Can you work these out from the drawing? Everything is in mm from the part's minimum corner. A direction names the side the tool comes from. Coordinates: 2 decimals unless noted, no trailing zeros. Order: outer loops, then holes, each group sorted by start corner. A loop starts at its lowest first (then second) coordinate and runs counter-clockwise, first axis right, second up. Notation, with made-up numbers: (19.25, 31.25) -> (56.25, 31.25) arc R19 cw to (56.25, 40.25) -> close; hole circle Ø3 at (16, 14). An arc over 180 degrees is marked (long way). Use a Markdown table: item, result. Add a question column.
1) If I drill on L1, parallel to Y at x = 70.8, z = 3.05; L2, parallel to Y at x = 70, z = 2; L3, parallel to Y at x = 69.5, z = 35.5, over which ranges is the centre line in solid material (lowest first)? Write a range as [from, to].
2) Which directions (+Z, -Z, +X, -X, +Y, -Y) give clear straight access to the entire face, cutting with the end or side of a thin tool? Please do the marked faces 1 and 2.
3) If we section it at C-C (x = 108): Write out the boundary of the cut face in (y, z), plus the area to 3 significant figures.
4) If we section it at D-D (z = 26): Write out the boundary of the cut face in (x, y).
5) If we section it at B-B (y = 10): Write out the boundary of the cut face in (x, z), plus the area to 3 significant figures.
6) If we section it at A-A (x = 70.8): Write out the boundary of the cut face in (y, z), plus the area to 3 significant figures.
7) Will these pins go through, and if not, where does the flat tip stop? pin 1 Ø7.5 at (x, y) = (113.79, 27.81) entering from +Z; pin 2 Ø4 at (x, y) = (10, 70.8) entering from -Z; pin 3 Ø10 at (x, z) = (65.5, 14.5) entering from -Y; pin 4 Ø10 at (y, z) = (80.5, 36) entering from -X.
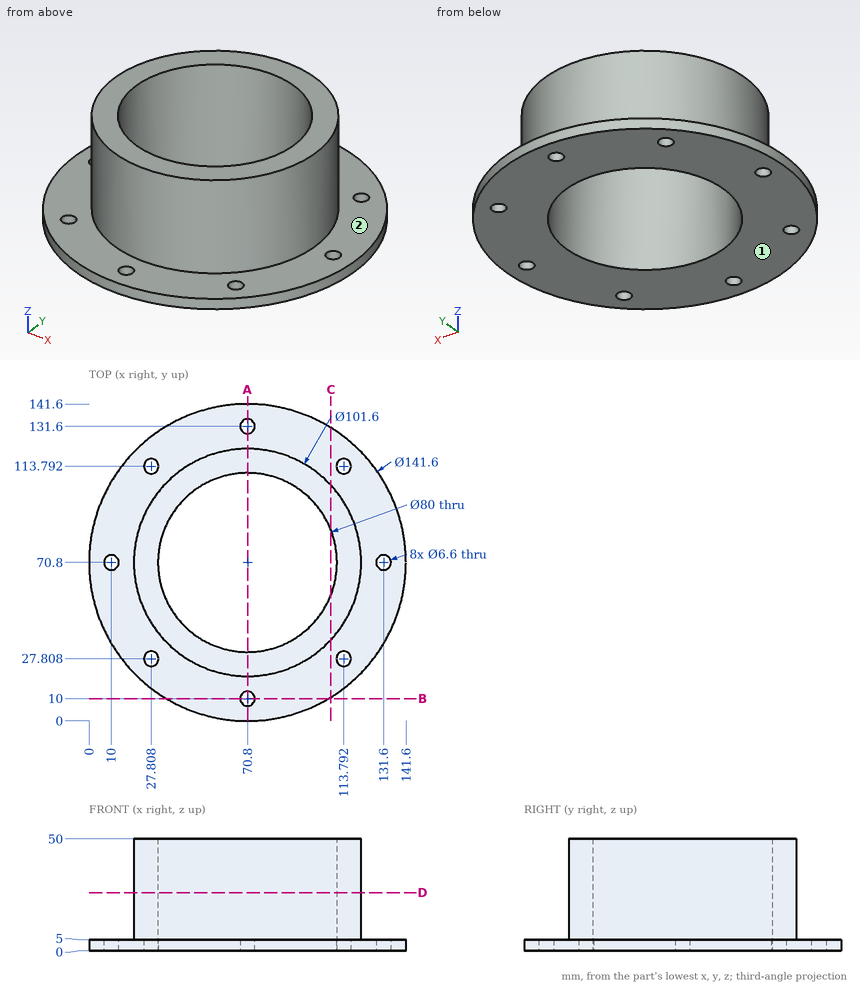
Answer sheet:
| question | item | result |
|---|---|---|
| 1 | L1 | [0, 6.7], [13.3, 30.8], [110.8, 128.3], [134.9, 141.6] |
| 1 | L2 | [0, 6.8], [13.2, 30.81], [110.79, 128.4], [134.8, 141.6] |
| 1 | L3 | [20.02, 30.82], [110.78, 121.58] |
| 2 | face 1 | -Z, +X, -X, +Y, -Y |
| 2 | face 2 | +Z |
| 3 | outline | (10.56, 0) -> (56.1, 0) -> (56.1, 50) -> (36.21, 50) -> (36.21, 5) -> (10.56, 5) -> close; (85.5, 0) -> (131.04, 0) -> (131.04, 5) -> (105.39, 5) -> (105.39, 50) -> (85.5, 50) -> close |
| 3 | area | 2,250 mm2 |
| 4 | outline | circle Ø101.6 at (70.8, 70.8); hole circle Ø80 at (70.8, 70.8) |
| 5 | outline | (34.52, 0) -> (67.5, 0) -> (67.5, 5) -> (34.52, 5) -> close; (74.1, 0) -> (107.08, 0) -> (107.08, 5) -> (74.1, 5) -> close |
| 5 | area | 330 mm2 |
| 6 | outline | (0, 0) -> (6.7, 0) -> (6.7, 5) -> (0, 5) -> close; (13.3, 0) -> (30.8, 0) -> (30.8, 50) -> (20, 50) -> (20, 5) -> (13.3, 5) -> close; (110.8, 0) -> (128.3, 0) -> (128.3, 5) -> (121.6, 5) -> (121.6, 50) -> (110.8, 50) -> close; (134.9, 0) -> (141.6, 0) -> (141.6, 5) -> (134.9, 5) -> close |
| 6 | area | 1,210 mm2 |
| 7 | pin 1 | z = 5 |
| 7 | pin 2 | through |
| 7 | pin 3 | y = 20 |
| 7 | pin 4 | x = 20.22 |
